CAD build for the part. Positions are in the model's coordinates, mm. Face numbers are marked on the shaded views. A direction names the side the tool comes from. Round coordinates to 2 decimals unless told otherwise and drop trailing zeros. Loops run counter-clockwise (first coordinate to the right, second up) from the corner with the lowest first, then second, coordinate; pieces in that order, holes last. Notation, with made-up numbers: M -7.75,51.25 L -0.75,51.25 A21 ccw -0.75,55.25 Z; hole C 62,-36 d5. An arc over 180 degrees is marked long. Use a Markdown table: item, result. Add a question column.
(1) Band-saw the part on B-B, the plane x = 8. Write the cut outline in (y, z), and give its area (3 significant figures).
(2) Flat gauge pins, fed straight in: P1, Ø0.5, axis at x = -0.5, y = 13, coming from the +Z side; P2, Ø3, axis at x = 7, y = 28, coming from the +Z side; P3, Ø3, axis at y = 30.5, z = -8, coming from the -X side. Where does each tip first touch, or does it go through?
(3) Band-saw the part on C-C, the plane y = 43. Write the cut outline in (x, z), and give its area (3 significant figures).
(4) Two-plate mould, pull along Y, no slides. Class the marked faces 1, 2 and 3: released by +Y, released by -Y, zero draft, split by the parting line, or undercut.
(5) Which spindle directions (+Z, -Z, +X, -X, +Y, -Y) get a long thin tool onto all of the face, cutting with end or side? Do the marked faces 4, 5 and 6. Say none if no direction does.
(6) Wall check: L1, parallel to Y at x = 7, z = -1.2; L2, parallel to Y at x = 7, z = -6.5; L3, parallel to Y at x = 5, z = -7.75. Give the ranges that are in metal, low to high.
(7) Band-saw the part on A-A, the plane y = 28. Write the cut outline in (x, z), and give its area (3 significant figures).
(8) Band-saw the part on D-D, the plane x = 12. Write the cut outline in (y, z), and give its area (3 significant figures).
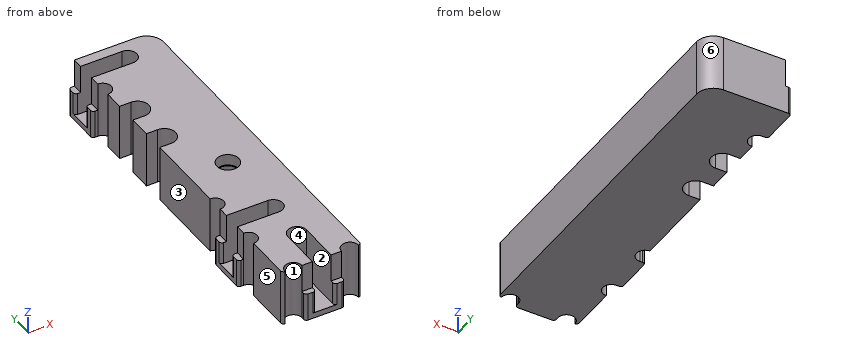
from build123d import *

# Parameters (mm, degrees)
SKETCH4_W           = 10
SKETCH4_H           = 62
BOSS_EXTRUDE1_DEPTH = 14
SKETCH10_W          = 1
SKETCH10_H          = 7
SKETCH10_W_2        = 7
SKETCH10_H_2        = 1
BOSS_EXTRUDE2_DEPTH = 5
CUT_EXTRUDE2_DEPTH  = 65.342831769
CUT_EXTRUDE6_DEPTH  = 65.342831769
SKETCH11_R          = 1.75
CUT_EXTRUDE7_DEPTH  = 8.5
SKETCH12_R          = 1.95
CUT_EXTRUDE8_DEPTH  = 2
CUT_EXTRUDE9_DEPTH  = 9
FILLET1_R           = 3
FILLET3_R           = 0.5


with BuildPart() as part:
    # Sketch4 → Boss-Extrude1 (new body)
    with BuildSketch(Plane(origin=(0, 0, 0), x_dir=(0, 0, -1), z_dir=(1, 0, 0))):
        with Locations((5, 31)):
            Rectangle(SKETCH4_W, SKETCH4_H)
    extrude(amount=BOSS_EXTRUDE1_DEPTH)

    # Sketch10 → Boss-Extrude2 (add)
    with BuildSketch(Plane(origin=(0, 0, -10), x_dir=(-1, 0, 0), z_dir=(0, 0, -1))):
        with Locations((0.5, 15)):
            Rectangle(SKETCH10_W, SKETCH10_H)
        with Locations((0.5, 58.5)):
            Rectangle(SKETCH10_W, SKETCH10_H)
        with Locations((-7, -0.5)):
            Rectangle(SKETCH10_W_2, SKETCH10_H_2)
    extrude(amount=-BOSS_EXTRUDE2_DEPTH)

    # Sketch5 → Cut-Extrude2 (cut, through all)
    with BuildSketch(Plane.XY):
        with BuildLine():
            Line((2, 44.5), (0, 44.5))
            Line((0, 44.5), (0, 48.5))
            Line((0, 48.5), (2, 48.5))
            ThreePointArc((2, 48.5), (4, 46.5), (2, 44.5))
        make_face()
        with BuildLine():
            Line((2, 36.5), (0, 36.5))
            Line((0, 36.5), (0, 40.5))
            Line((0, 40.5), (2, 40.5))
            ThreePointArc((2, 40.5), (4, 38.5), (2, 36.5))
        make_face()
    extrude(amount=-CUT_EXTRUDE2_DEPTH, mode=Mode.SUBTRACT)

    # Sketch9 → Cut-Extrude6 (cut, through all)
    with BuildSketch(Plane.XY):
        with BuildLine():
            Line((0, 52), (-1, 52))
            ThreePointArc((-1, 52), (-2.5, 53.5), (-1, 55))
            Line((-1, 55), (0, 55))
            ThreePointArc((0, 55), (1.5, 53.5), (0, 52))
        make_face()
        with BuildLine():
            Line((0, 18.5), (-1, 18.5))
            ThreePointArc((-1, 18.5), (-2.5, 20), (-1, 21.5))
            Line((-1, 21.5), (0, 21.5))
            ThreePointArc((0, 21.5), (1.5, 20), (0, 18.5))
        make_face()
        with BuildLine():
            Line((0, 8.5), (-1, 8.5))
            ThreePointArc((-1, 8.5), (-2.5, 10), (-1, 11.5))
            Line((-1, 11.5), (0, 11.5))
            ThreePointArc((0, 11.5), (1.5, 10), (0, 8.5))
        make_face()
        with BuildLine():
            Line((0.5, -1), (0.5, 0))
            ThreePointArc((0.5, 0), (2, 1.5), (3.5, 0))
            Line((3.5, 0), (3.5, -1))
            ThreePointArc((3.5, -1), (2, -2.5), (0.5, -1))
        make_face()
        with BuildLine():
            Line((13.5, 0), (13.5, -1))
            ThreePointArc((13.5, -1), (12, -2.5), (10.5, -1))
            Line((10.5, -1), (10.5, 0))
            ThreePointArc((10.5, 0), (12, 1.5), (13.5, 0))
        make_face()
    extrude(amount=-CUT_EXTRUDE6_DEPTH, mode=Mode.SUBTRACT)

    # Sketch11 → Cut-Extrude7 (cut)
    with BuildSketch(Plane.XY):
        with Locations((7, 28)):
            Circle(SKETCH11_R)
    extrude(amount=-CUT_EXTRUDE7_DEPTH, mode=Mode.SUBTRACT)

    # Sketch12 → Cut-Extrude8 (cut)
    with BuildSketch(Plane.XY):
        with Locations((7, 28)):
            Circle(SKETCH12_R)
    extrude(amount=-CUT_EXTRUDE8_DEPTH, mode=Mode.SUBTRACT)

    # Sketch13 → Cut-Extrude9 (cut)
    with BuildSketch(Plane.XY):
        with BuildLine():
            Line((8.65, 7.35), (8.65, -1))
            ThreePointArc((8.65, -1), (7, -2.65), (5.35, -1))
            Line((5.35, -1), (5.35, 7.35))
            ThreePointArc((5.35, 7.35), (7, 9), (8.65, 7.35))
        make_face()
        with BuildLine():
            Line((7.35, 13.35), (-1, 13.35))
            ThreePointArc((-1, 13.35), (-2.65, 15), (-1, 16.65))
            Line((-1, 16.65), (7.35, 16.65))
            ThreePointArc((7.35, 16.65), (9, 15), (7.35, 13.35))
        make_face()
        with BuildLine():
            Line((7.35, 56.85), (-1, 56.85))
            ThreePointArc((-1, 56.85), (-2.65, 58.5), (-1, 60.15))
            Line((-1, 60.15), (7.35, 60.15))
            ThreePointArc((7.35, 60.15), (9, 58.5), (7.35, 56.85))
        make_face()
    extrude(amount=-CUT_EXTRUDE9_DEPTH, mode=Mode.SUBTRACT)

    # Fillet1
    fillet1_edges = [part.edges().sort_by_distance(p)[0] for p in [
        (14, 62, -5),
    ]]
    fillet(fillet1_edges, radius=FILLET1_R)

    # Fillet3
    fillet3_edges = [part.edges().sort_by_distance(p)[0] for p in [
        (14, 0, -5),
        (0, 0, -5),
        (-1, 55, -7.5),
        (-1, 62, -7.5),
        (-1, 18.5, -7.5),
        (-1, 11.5, -7.5),
        (3.5, -1, -7.5),
        (10.5, -1, -7.5),
        (-1, 56.85, -7),
        (-1, 60.15, -7),
        (-1, 13.35, -7),
        (-1, 16.65, -7),
        (5.35, -1, -7),
        (8.65, -1, -7),
    ]]
    fillet(fillet3_edges, radius=FILLET3_R - 0.0001)  # a hair under: the kernel refuses the full size


solid = part.part
Return value:
| question | item | result |
|---|---|---|
| 1 | outline | M -1,-10 L 62,-10 L 62,0 L 60.02,0 L 60.02,-9 L 56.98,-9 L 56.98,0 L 29.67,0 L 29.67,-2 L 29.44,-2 L 29.44,-8.5 L 26.56,-8.5 L 26.56,-2 L 26.33,-2 L 26.33,0 L 16.52,0 L 16.52,-9 L 13.48,-9 L 13.48,0 L 8.66,0 L 8.66,-9 L -1,-9 Z |
| 1 | area | 463 mm^2 |
| 2 | P1 | z = -5 |
| 2 | P2 | z = -8.5 |
| 2 | P3 | x = 0 |
| 3 | outline | M 0,-10 L 14,-10 L 14,0 L 0,0 Z |
| 3 | area | 140 mm^2 |
| 4 | face 1 | released by -Y |
| 4 | face 2 | zero draft |
| 4 | face 3 | undercut |
| 5 | face 4 | +Z, -Y |
| 5 | face 5 | +Z, -Z, -X, -Y |
| 5 | face 6 | +Z, -Z, +X, +Y |
| 6 | L1 | 9 to 13.35, 16.65 to 26.05, 29.95 to 56.85, 60.15 to 62 |
| 6 | L2 | 9 to 13.35, 16.65 to 26.25, 29.75 to 56.85, 60.15 to 62 |
| 6 | L3 | -0.98 to 13.35, 16.65 to 56.85, 60.15 to 62 |
| 7 | outline | M 0,-10 L 14,-10 L 14,0 L 8.95,0 L 8.95,-2 L 8.75,-2 L 8.75,-8.5 L 5.25,-8.5 L 5.25,-2 L 5.05,-2 L 5.05,0 L 0,0 Z |
| 7 | area | 109 mm^2 |
| 8 | outline | M 1.5,-10 L 61.83,-10 L 61.83,0 L 1.5,0 Z |
| 8 | area | 603 mm^2 |
